Geometry check sheet. Reference: the model listing, model coordinates, mm. Face numbers are marked on the shaded views. A direction names the side the tool comes from. Round coordinates to 2 decimals unless told otherwise and drop trailing zeros. Loops run counter-clockwise (first coordinate to the right, second up) from the corner with the lowest first, then second, coordinate; pieces in that order, holes last. Notation, with made-up numbers: (21.25, 41.25) -> (71.25, 41.25) arc R10 ccw to (71.25, 45.25) -> close; hole circle Ø5 at (6.5, 80). An arc over 180 degrees is marked (long way). Use one line per item in the form item = value.
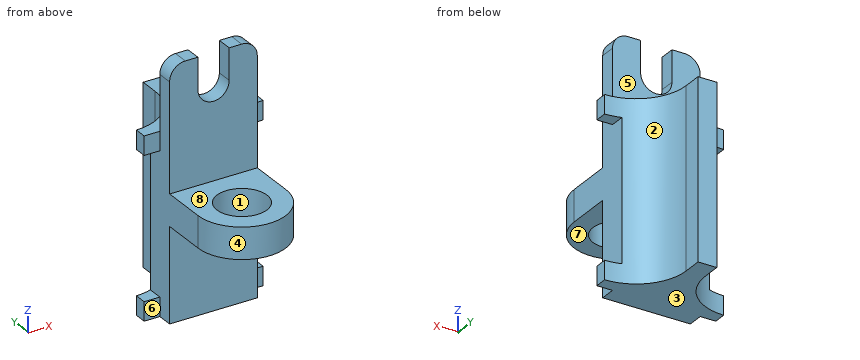
from build123d import *

# Parameters (mm, degrees)
BOSS_EXTRUDE3_DEPTH      = 89
BOSS_EXTRUDE3_DEPTH_BACK = 70
SKETCH7_W                = 56
SKETCH7_H                = 10
BOSS_EXTRUDE4_DEPTH      = 44
BOSS_EXTRUDE4_DEPTH_BACK = 70
BOSS_EXTRUDE5_DEPTH      = 10
BOSS_EXTRUDE5_DEPTH_BACK = 10
SKETCH1_R                = 16
CUT_EXTRUDE1_REACH       = 131.484
FILLET1_R                = 10
CUT_EXTRUDE3_REACH       = 131.484
SKETCH10_W               = 10
SKETCH10_H               = 90


with BuildPart() as part:
    # Sketch7 → Boss-Extrude3 (new, two sides: drawn at the far end of the back side and taken through both)
    with BuildSketch(Plane.XY.offset(-BOSS_EXTRUDE3_DEPTH_BACK)):
        with Locations((28, 34)):
            Rectangle(SKETCH7_W, SKETCH7_H)
    extrude(amount=BOSS_EXTRUDE3_DEPTH + BOSS_EXTRUDE3_DEPTH_BACK)

    # Sketch5 → Boss-Extrude4 (add, two sides: drawn at the far end of the back side and taken through both)
    with BuildSketch(Plane.XY.offset(-BOSS_EXTRUDE4_DEPTH_BACK)):
        with BuildLine():
            Line((22, 79), (22, 91))
            Line((22, 91), (34, 91))
            Line((34, 91), (34, 79))
            ThreePointArc((34, 79), (43.372583002, 56.372583002), (66, 47))
            Line((66, 47), (66, 39))
            Line((66, 39), (-10, 39))
            Line((-10, 39), (-10, 47))
            ThreePointArc((-10, 47), (12.627416998, 56.372583002), (22, 79))
        make_face()
    extrude(amount=BOSS_EXTRUDE4_DEPTH + BOSS_EXTRUDE4_DEPTH_BACK)

    # Sketch1 → Boss-Extrude5 (add, two sides: drawn at the far end of the back side and taken through both)
    with BuildSketch(Plane.XY.offset(-BOSS_EXTRUDE5_DEPTH_BACK)):
        with BuildLine():
            Line((0, 0), (0, 29))
            Line((0, 29), (56, 29))
            Line((56, 29), (56, 0))
            ThreePointArc((56, 0), (28, -28), (0, 0))
        make_face()
        with Locations((28, 0)):
            Circle(SKETCH1_R, mode=Mode.SUBTRACT)
    extrude(amount=BOSS_EXTRUDE5_DEPTH + BOSS_EXTRUDE5_DEPTH_BACK)

    # Sketch9 → Cut-Extrude1 (cut, up to next)
    with BuildSketch(Plane(origin=(0, 39, 0), x_dir=(1, 0, 0), z_dir=(0, 1, 0)), mode=Mode.PRIVATE) as cut_extrude1_sk1:
        with BuildLine():
            Line((38.033469933, -69), (38.033469933, -89))
            Line((38.033469933, -89), (18.033469933, -89))
            Line((18.033469933, -89), (18.033469933, -69))
            ThreePointArc((18.033469933, -69), (28.033469933, -59), (38.033469933, -69))
        make_face()
    cut_extrude1_tool1 = extrude(cut_extrude1_sk1.sketch, amount=-CUT_EXTRUDE1_REACH, mode=Mode.PRIVATE) & part.part
    add(cut_extrude1_tool1.solids().sort_by_distance((28.03347, 39, 74.983585))[0], mode=Mode.SUBTRACT)

    # Fillet1
    fillet1_edges = [part.edges().sort_by_distance(p)[0] for p in [
        (56, 34, 89),
        (0, 34, 89),
    ]]
    fillet(fillet1_edges, radius=FILLET1_R)

    # Sketch10 → Cut-Extrude3 (cut, up to next)
    with BuildSketch(Plane.XZ.offset(-39), mode=Mode.PRIVATE) as cut_extrude3_sk1:
        with Locations((-5, -13)):
            Rectangle(SKETCH10_W, SKETCH10_H)
    cut_extrude3_tool1 = extrude(cut_extrude3_sk1.sketch, amount=-CUT_EXTRUDE3_REACH, mode=Mode.PRIVATE) & part.part
    # Sketch10 → Cut-Extrude3 (cut, up to next)
    with BuildSketch(Plane.XZ.offset(-39), mode=Mode.PRIVATE) as cut_extrude3_sk2:
        with Locations((61, -13)):
            Rectangle(SKETCH10_W, SKETCH10_H)
    cut_extrude3_tool2 = extrude(cut_extrude3_sk2.sketch, amount=-CUT_EXTRUDE3_REACH, mode=Mode.PRIVATE) & part.part
    add(cut_extrude3_tool1.solids().sort_by_distance((-5, 39, -13))[0], mode=Mode.SUBTRACT)
    add(cut_extrude3_tool2.solids().sort_by_distance((61, 39, -13))[0], mode=Mode.SUBTRACT)


solid = part.part
1. Material ranges on line 1 along Y through (x, z) = (28, 3); line 2 along Z through (x, y) = (32.5, 47); line 3 along Y through (x, z) = (42.5, 70), recorded low to high.
Return value:
line_1 = -28 to -16, 16 to 91
line_2 = -70 to 44
line_3 = 29 to 39
2. Gauge pin test, flat ends, axial feed: pin 1 (3 mm diameter, centred on x = 63, y = 46, fed in from +Z); pin 2 (3 mm diameter, centred on x = 20, y = -15, fed in from +Z); pin 3 (1.5 mm diameter, centred on x = 9, z = 8.5, fed in from +Y); pin 4 (19 mm diameter, centred on x = 28, y = 0, fed in from -Z). Record the tip position at first contact, or that the pin passes through.
Return value:
pin_1 = 44
pin_2 = 10
pin_3 = 53.82
pin_4 = through
3. Section check B-B (x = 25.5). Record the boundary of the cut face in (y, z).
Return value:
outline = (-27.89, -10) -> (-15.8, -10) -> (-15.8, 10) -> (-27.89, 10) -> close; (15.8, -10) -> (29, -10) -> (29, -70) -> (91, -70) -> (91, 44) -> (39, 44) -> (39, 59.33) -> (29, 59.33) -> (29, 10) -> (15.8, 10) -> close
4. Mould release check, pull along X, two halves, no side actions. Record for the marked faces 1, 2, 3 and 4: released by +X, released by -X, zero draft, split by the parting line, or undercut.
Return value:
face_1 = undercut
face_2 = released by +X
face_3 = zero draft
face_4 = split by the parting line
5. Section check D-D (z = 66). Record the boundary of the cut face in (x, y), then the cut area to 3 significant figures.
Return value:
outline = (0, 29) -> (18.49, 29) -> (18.49, 39) -> (0, 39) -> close; (37.57, 29) -> (56, 29) -> (56, 39) -> (37.57, 39) -> close
area = 369 mm2
6. Section check A-A (y = 7). Record the boundary of the cut face in (x, z), then the cut area to 4 significant figures.
Return value:
outline = (0, -10) -> (13.61, -10) -> (13.61, 10) -> (0, 10) -> close; (42.39, -10) -> (56, -10) -> (56, 10) -> (42.39, 10) -> close
area = 544.5 mm2
7. Section check C-C (z = -53.5). Record the boundary of the cut face in (x, y), then the cut area to 3 significant figures.
Return value:
outline = (0, 29) -> (56, 29) -> (56, 48.6) arc R32 cw to (34, 79) -> (34, 91) -> (22, 91) -> (22, 79) arc R32 cw to (0, 48.6) -> close
area = 1,960 mm2
8. Tool access check on the marked faces 5, 6, 7 and 8. Record the directions out of +Z, -Z, +X, -X, +Y, -Y that give a thin tool (end or side, any length) a straight path to the whole face; none if there is none.
Return value:
face_5 = +Z, +X, -X, +Y
face_6 = +Z, -Z, -X, -Y
face_7 = -Z, +X, -X, -Y
face_8 = +Z, +X, -X, -Y
